Part model, mm, in its own coordinate system. A direction names the side the tool comes from. Round coordinates to 2 decimals unless told otherwise and drop trailing zeros. Loops run counter-clockwise (first coordinate to the right, second up) from the corner with the lowest first, then second, coordinate; pieces in that order, holes last. Notation, with made-up numbers: M -28.75,-23.5 L -0.75,-23.5 A13 ccw -0.75,0.5 Z; hole C 16,54.25 d11. An arc over 180 degrees is marked long. Put each result on its own line as item: value. Start each with the question number.
1) Which spindle directions (+Z, -Z, +X, -X, +Y, -Y) get a long thin tool onto all of the face, cutting with end or side? Do faces 1 (the flat face through (75, 0, 29)), 2 (the cylindrical face through (-27.203, 2.436, -8.51)). Say none if no direction does.
2) Pull direction Z, two halves, no side cores. Call faces 3 (the flat face through (-1, -3.175, -11)), 4 (the cylindrical face through (-58.648, 0.044, -62.274)), 5 (the flat face through (-1, 0, 50.8)): +Z half, -Z half, draft (parallel to the pull), parting line (faces both ways), or undercut.
3) Drop a flat-ended pin along its axis: pin 1 Ø3 at (x, z) = (0, -60.8) entering from +Y. Give the stop position or say it passes through.
4) Slice it at A-A on z = 29.2. Give the cut face in (x, y) (3 decimals).
5) Probe line 1 along X through (y, z) = (0.25, -60.8); line 2 along X through (y, z) = (-1.75, -5.8); line 3 along X through (y, z) = (1.5, -17.8). List the from-to ranges inside material, lowest first.
6) Slice it at C-C on y = -1. State how many separate pieces and enclosed holes the cut face has, then the cut area to 3 significant figures.
7) Slice it at D-D on x = 67. Give the cut face in (y, z) (3 decimals), then the cut area to 3 significant figures.
8) Slice it at B-B on x = 31.9. Give the cut face in (y, z) (3 decimals), then the cut area to 3 significant figures.
```python
from build123d import *

# Parameters (mm, degrees)
CROQUIS1_W              = 150
CROQUIS1_H              = 101.6
SALIENTE_EXTRUIR1_DEPTH = 3.175
CROQUIS2_R              = 2
CROQUIS2_R_2            = 11
CROQUIS2_R_3            = 1.5
CROQUIS2_R_4            = 6.35
CORTAR_EXTRUIR1_DEPTH   = 91.807282197
REDONDEO1_R             = 6.35
CROQUIS3_R              = 1.5
CORTAR_EXTRUIR2_DEPTH   = 91.807282197
CORTAR_EXTRUIR3_START   = 3.175
CROQUIS4_R              = 12.5
CORTAR_EXTRUIR3_DEPTH   = 1.5
CROQUIS9_R              = 2.5
CORTAR_EXTRUIR6_DEPTH   = 91.807282197
CHAFL_N1_SIZE           = 2.5
CROQUIS10_W             = 150
CROQUIS10_H             = 20
CROQUIS10_R             = 2
SALIENTE_EXTRUIR2_DEPTH = 6.35


with BuildPart() as part:
    # Croquis1 → Saliente-Extruir1 (new, symmetric)
    with BuildSketch(Plane(origin=(0, 0, 0), x_dir=(1, 0, 0), z_dir=(0, 1, 0))):
        Rectangle(CROQUIS1_W, CROQUIS1_H)
    extrude(amount=SALIENTE_EXTRUIR1_DEPTH, both=True)

    # Croquis2 → Cortar-Extruir1 (cut, through all)
    with BuildSketch(Plane(origin=(0, 3.175, 0), x_dir=(1, 0, 0), z_dir=(0, 1, 0))):
        with Locations(Location((67, 40.8, 0), (0, 0, 270))):
            Circle(CROQUIS2_R)
        with Locations(Location((67, -29.2, 0), (0, 0, 90))):
            Circle(CROQUIS2_R)
        with Locations(Location((-15, 5.8, 0), (0, 0, 270))):
            Circle(CROQUIS2_R_2)
        with Locations(Location((-67.25, 5.8, 0), (0, 0, 270))):
            Circle(CROQUIS2_R_3)
        with Locations(Location((31.9, 5.8, 0), (0, 0, 270))):
            Circle(CROQUIS2_R_4)
        with Locations((69.9, 5.8)):
            Circle(CROQUIS2_R_4)
    extrude(amount=-CORTAR_EXTRUIR1_DEPTH, mode=Mode.SUBTRACT)

    # Redondeo1
    redondeo1_edges = [part.edges().sort_by_distance(p)[0] for p in [
        (75, 0, -2.016813512),
        (75, 0, -9.583186488),
    ]]
    fillet(redondeo1_edges, radius=REDONDEO1_R)

    # Croquis3 → Cortar-Extruir2 (cut, through all)
    with BuildSketch(Plane(origin=(0, 3.175, 0), x_dir=(1, 0, 0), z_dir=(0, 1, 0))):
        with Locations(Location((-15, -9.2, 0), (0, 0, 270))):
            Circle(CROQUIS3_R)
        with Locations(Location((-15, -18.2, 0), (0, 0, 270))):
            Circle(CROQUIS3_R)
        with Locations(Location((-27.990381057, 13.3, 0), (0, 0, 270))):
            Circle(CROQUIS3_R)
        with Locations(Location((-35.784609691, 17.8, 0), (0, 0, 270))):
            Circle(CROQUIS3_R)
        with Locations(Location((-2.009618943, 13.3, 0), (0, 0, 270))):
            Circle(CROQUIS3_R)
        with Locations(Location((5.784609691, 17.8, 0), (0, 0, 270))):
            Circle(CROQUIS3_R)
    extrude(amount=-CORTAR_EXTRUIR2_DEPTH, mode=Mode.SUBTRACT)

    # Croquis4 → Cortar-Extruir3 (cut)
    with BuildSketch(Plane(origin=(0, 0, 0), x_dir=(1, 0, 0), z_dir=(0, 1, 0)).offset(CORTAR_EXTRUIR3_START)):
        with Locations(Location((-15, 5.8, 0), (0, 0, 270))):
            Circle(CROQUIS4_R)
    extrude(amount=-CORTAR_EXTRUIR3_DEPTH, mode=Mode.SUBTRACT)

    # Croquis9 → Cortar-Extruir6 (cut, through all)
    with BuildSketch(Plane(origin=(0, 3.175, 0), x_dir=(1, 0, 0), z_dir=(0, 1, 0))):
        with Locations(Location((3.5, 5.8, 0), (0, 0, 270))):
            Circle(CROQUIS9_R)
        with Locations(Location((-33.5, 5.8, 0), (0, 0, 90))):
            Circle(CROQUIS9_R)
    extrude(amount=-CORTAR_EXTRUIR6_DEPTH, mode=Mode.SUBTRACT)

    # Chaflán1
    chafl_n1_edges = [part.edges().sort_by_distance(p)[0] for p in [
        (3.5, 3.175, -8.3),
        (-33.5, 3.175, -3.3),
    ]]
    chamfer(chafl_n1_edges, length=CHAFL_N1_SIZE)

    # Croquis10 → Saliente-Extruir2 (add)
    with BuildSketch(Plane(origin=(0, 3.175, 0), x_dir=(1, 0, 0), z_dir=(0, 1, 0))):
        with Locations((0, 60.8)):
            Rectangle(CROQUIS10_W, CROQUIS10_H)
        with Locations(Location((0, 60.8, 0), (0, 0, 270))):
            Circle(CROQUIS10_R, mode=Mode.SUBTRACT)
        with Locations(Location((-60, 60.8, 0), (0, 0, 270))):
            Circle(CROQUIS10_R, mode=Mode.SUBTRACT)
        with Locations(Location((60, 60.8, 0), (0, 0, 270))):
            Circle(CROQUIS10_R, mode=Mode.SUBTRACT)
    extrude(amount=-SALIENTE_EXTRUIR2_DEPTH)


solid = part.part
```
Recorded:
1. face 1: +Z, -Z, +X, +Y, -Y
1. face 2: +Y
2. face 3: draft
2. face 4: undercut
2. face 5: +Z half
3. pin 1: passes through
4. outline: M -75,-3.175 L 65,-3.175 L 65,3.175 L -75,3.175 Z; M 69,-3.175 L 75,-3.175 L 75,3.175 L 69,3.175 Z
5. line 1: x = -75 to -62, -58 to -2, 2 to 58, 62 to 75
5. line 2: x = -75 to -68.75, -65.75 to -36, -31 to -26, -4 to 1, 6 to 25.55, 38.25 to 63.55
5. line 3: x = -75 to -37.28, -34.28 to 4.28, 7.28 to 74.97
6. separate pieces: 1
6. enclosed holes: 16
6. area: 17,400 mm2
7. outline: M -3.175,-70.8 L 3.175,-70.8 L 3.175,-42.8 L -3.175,-42.8 Z; M -3.175,-38.8 L 3.175,-38.8 L 3.175,-11.449 L -3.175,-11.449 Z; M -3.175,-0.151 L 3.175,-0.151 L 3.175,27.2 L -3.175,27.2 Z; M -3.175,31.2 L 3.175,31.2 L 3.175,50.8 L -3.175,50.8 Z
7. area: 650 mm2
8. outline: M -3.175,-70.8 L 3.175,-70.8 L 3.175,-12.15 L -3.175,-12.15 Z; M -3.175,0.55 L 3.175,0.55 L 3.175,50.8 L -3.175,50.8 Z
8. area: 692 mm2
